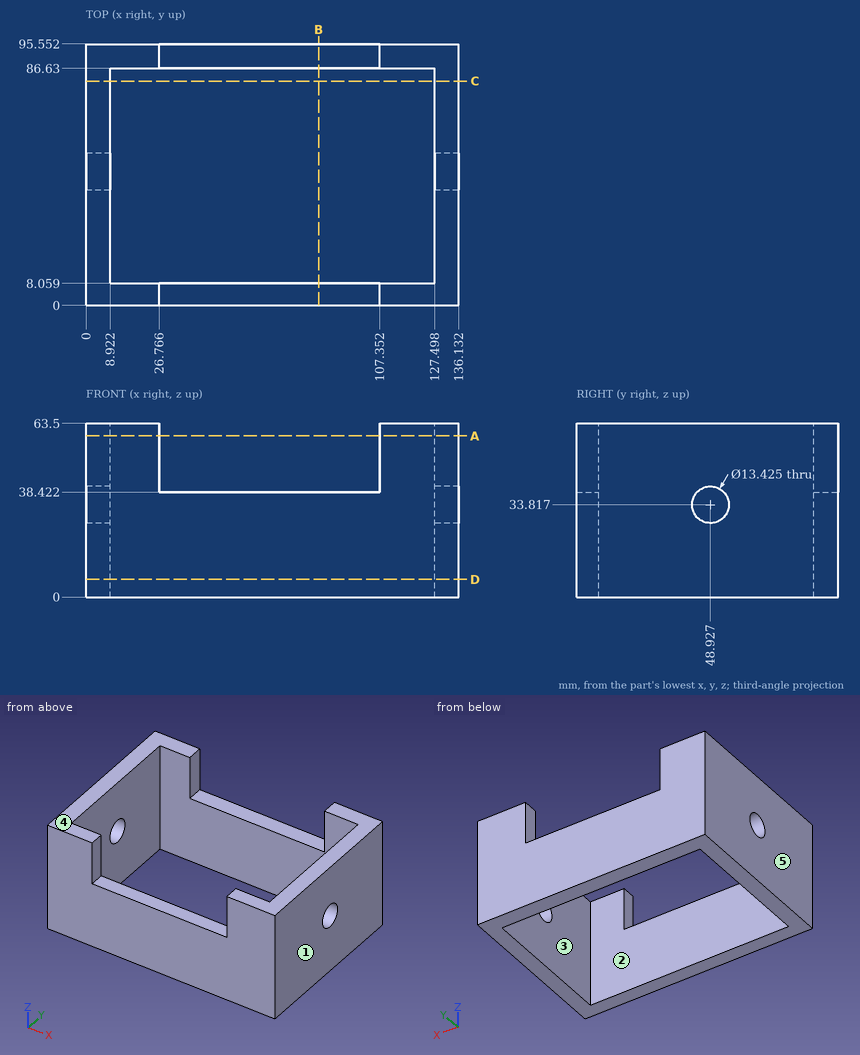
Answer from the drawing. Dimensions are ordinates in mm from the lowest x, y and z of the part. A direction names the side the tool comes from. Give positions to 0.01 mm unless a question says otherwise; leave off trailing zeros. Loops run counter-clockwise (first coordinate to the right, second up) from the corner with the lowest first, then second, coordinate; pieces in that order, holes last. Notation, with made-up numbers: (8.25, -1) - (48.25, -1) arc R17 cw to (48.25, 4) - close; hole circle Ø4 at (-8, 65). An arc over 180 degrees is marked (long way). Answer as CSV lines item,"result". Start each with the question number.
Item 1: A cutting plane is placed at A-A on z = 59. Determine the outline of the cut face in (x, y) (1 decimal), then the cut area to 3 significant figures.
Item 2: The mould has two halves that part along X. Classify the marked faces 3, 4 and 5: +X half, -X half, draft (parallel to the pull), parting line (faces both ways), or undercut.
Item 3: For the marked faces 1 and 2, determine the directions among +Z, -Z, +X, -X, +Y, -Y from which every point of the face is accessible in a straight line to the end or side of a thin tool.
Item 4: A cutting plane is placed at C-C on y = 82. Determine the outline of the cut face in (x, z), then the cut area to 4 significant figures.
Item 5: A cutting plane is placed at D-D on z = 6.5. Determine the outline of the cut face in (x, y).
Item 6: A cutting plane is placed at B-B on x = 85. Determine the outline of the cut face in (y, z).
Item 7: Find the intervals of material crossed by line 1 (X direction, y = 20.5, z = 33); line 2 (Y direction, x = 34, z = 26.5); line 3 (X direction, y = 90, z = 61.5) (1 decimal), in increasing order. Write a range as from..to.
Item 8: Each of these flat-tipped pins is pushed along its axis until it touches: pin 1 (10 mm diameter, centred on x = 54.5, y = 91.5, fed in from +Z); pin 2 (17.5 mm diameter, centred on y = 48.93, z = 33.82, fed in from +X); pin 3 (8 mm diameter, centred on y = 48.93, z = 33.82, fed in from -X). Where does it stop, or does it pass through?
Found:
1,outline,"(0, 0) - (26.8, 0) - (26.8, 8.1) - (8.9, 8.1) - (8.9, 86.6) - (26.8, 86.6) - (26.8, 95.6) - (0, 95.6) - close; (107.4, 0) - (136.1, 0) - (136.1, 95.6) - (107.4, 95.6) - (107.4, 86.6) - (127.5, 86.6) - (127.5, 8.1) - (107.4, 8.1) - close"
1,area,"2,320 mm^2"
2,face 3,"undercut"
2,face 4,"draft"
2,face 5,"-X half"
3,face 1,"+Z, -Z, +X, +Y, -Y"
3,face 2,"+Z, -Z"
4,outline,"(0, 0) - (8.92, 0) - (8.92, 63.5) - (0, 63.5) - close; (127.5, 0) - (136.13, 0) - (136.13, 63.5) - (127.5, 63.5) - close"
4,area,"1,115 mm^2"
5,outline,"(0, 0) - (136.13, 0) - (136.13, 95.55) - (0, 95.55) - close; hole (8.92, 8.06) - (127.5, 8.06) - (127.5, 86.63) - (8.92, 86.63) - close"
6,outline,"(0, 0) - (8.06, 0) - (8.06, 38.42) - (0, 38.42) - close; (86.63, 0) - (95.55, 0) - (95.55, 38.42) - (86.63, 38.42) - close"
7,line 1,"x = 0..8.92, 127.5..136.13"
7,line 2,"y = 0..8.06, 86.63..95.55"
7,line 3,"x = 0..26.8, 107.4..136.1"
8,pin 1,"stops at z = 38.42"
8,pin 2,"stops at x = 136.13"
8,pin 3,"passes through"
